Could you check a few things on this drawing? It's one solid part, dimensions in mm from its lowest x, y, z. Give positions to 0.01 mm unless a question says otherwise; leave off trailing zeros. Loops run counter-clockwise (first coordinate to the right, second up) from the corner with the lowest first, then second, coordinate; pieces in that order, holes last. Notation, with made-up numbers: (-9, -32) - (49, -32) arc R5 ccw to (49, -23) - close; hole circle Ø1 at (3, 13). An arc over 180 degrees is marked (long way). Write item = value, one per line.
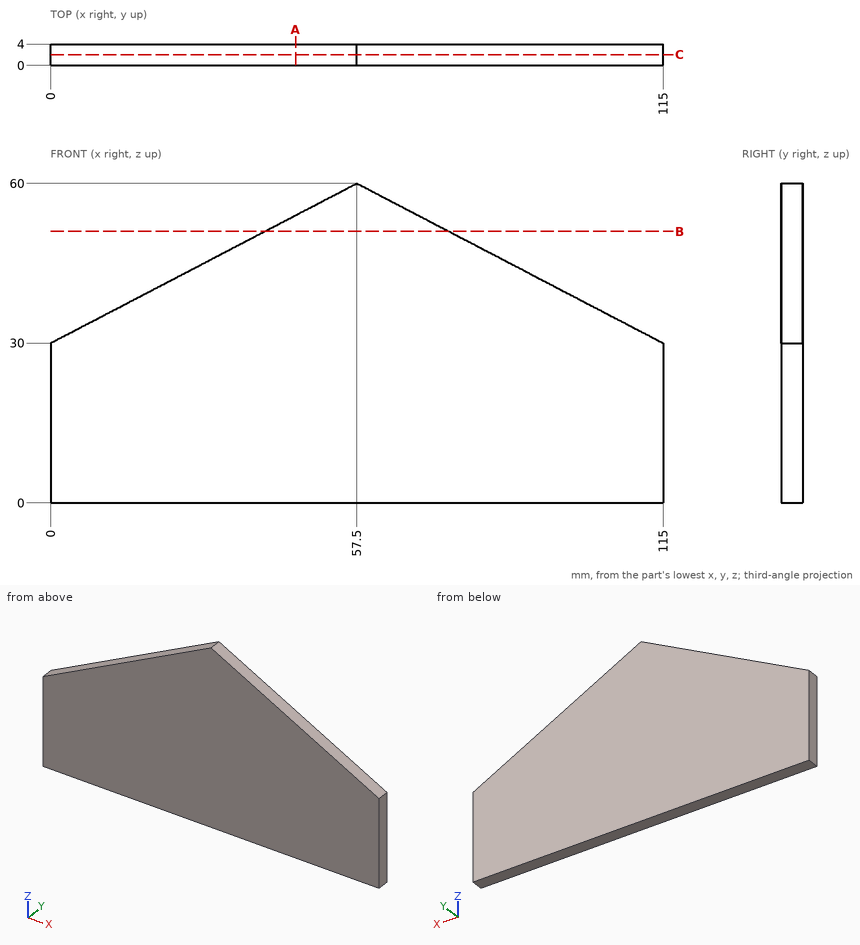
Q1. Imagine slicing it at A-A, the plane x = 46. Write out the boundary of the cut face in (y, z), then the cut area to 3 significant figures.
Output:
outline = (0, 0) - (4, 0) - (4, 54) - (0, 54) - close
area = 216 mm2
Q2. I need wall thicknesses on L1, parallel to Z at x = 32, y = 2.1; L2, parallel to Z at x = 18, y = 0.4; L3, parallel to X at y = 2.8, z = 31. Which ranges of each line are inside material? Lowest first, please.
Output:
L1 = 0 to 46.7
L2 = 0 to 39.39
L3 = 1.92 to 113.08
Q3. Imagine slicing it at B-B, the plane z = 51. Write out the boundary of the cut face in (x, y), then the cut area to 3 significant figures.
Output:
outline = (40.25, 0) - (74.75, 0) - (74.75, 4) - (40.25, 4) - close
area = 138 mm2
Q4. Imagine slicing it at C-C, the plane y = 2. Write out the boundary of the cut face in (x, z), then the cut area to 4 significant figures.
Output:
outline = (0, 0) - (115, 0) - (115, 30) - (57.5, 60) - (0, 30) - close
area = 5,175 mm2
